Check sheet for the drawn part. Datum: minimum x, y, z corner. Units: mm. A direction names the side the tool comes from. Coordinates: 2 decimals unless noted, no trailing zeros. Write each loop counter-clockwise with the first axis right and the second up, starting at its lowest first coordinate (ties: lowest second). Pieces come first, ordered by that corner, then holes. Notation, with made-up numbers: (22.5, 63) - (66.5, 63) arc R17 ccw to (66.5, 77) - close; hole circle Ø7 at (54, 61). An arc over 180 degrees is marked (long way). Answer as CSV lines item,"result". Start each with the question number.
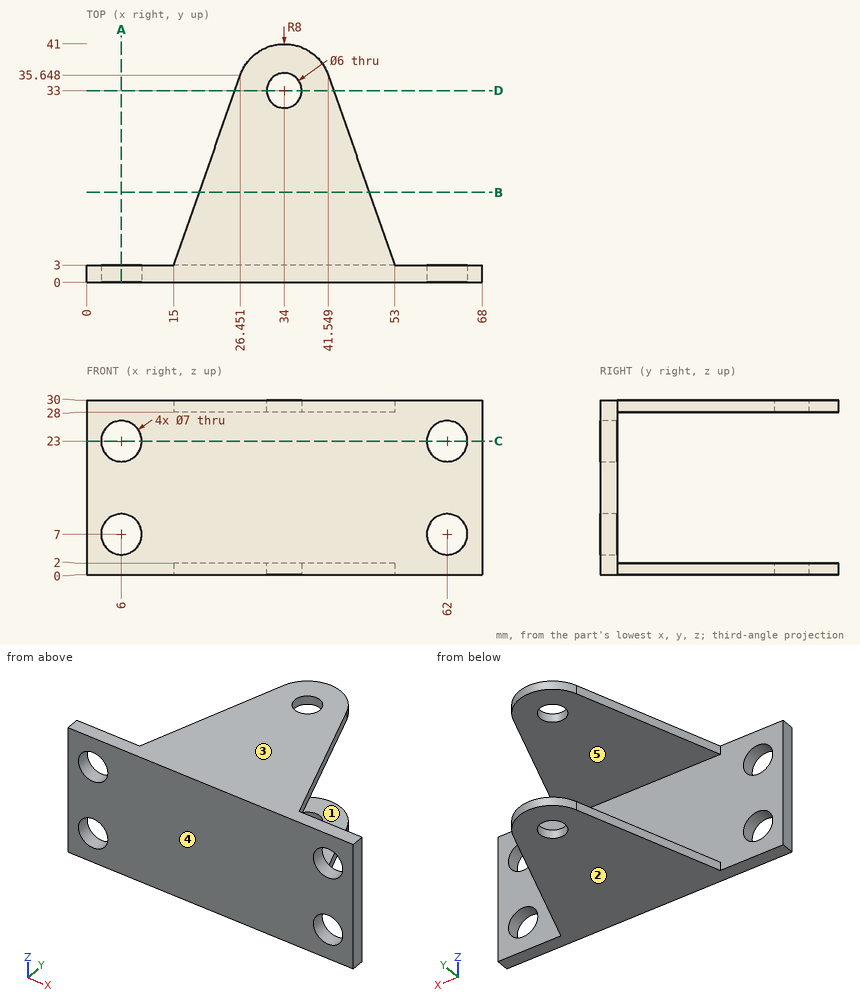
(1) Go/stop test with flat-tipped pins: P1, Ø1, axis at x = 8.5, z = 6.5, coming from the +Y side; P2, Ø8, axis at x = 62, z = 7, coming from the +Y side; P3, Ø12, axis at x = 43, z = 25.5, coming from the -Y side. Record where each tip stops, or that it passes through.
(2) Material ranges on probe 1 along X at (y, z) = (2.4, 23); probe 2 along Z at (x, y) = (30.5, 38); probe 3 along Y at (x, z) = (34, 28.4), recorded low to high. Write a range as from..to.
(3) Cross-section at D-D on y = 33. Record the boundary of the cut face in (x, z), plus the area to 3 significant figures.
(4) Cross-section at B-B on y = 15.5. Record the boundary of the cut face in (x, z).
(5) Tool access check on the marked faces 1 and 2. Record the directions out of +Z, -Z, +X, -X, +Y, -Y that give a thin tool (end or side, any length) a straight path to the whole face; none if there is none.
(6) Cross-section at C-C on z = 23. Record the boundary of the cut face in (x, y), plus the area to 3 significant figures.
(7) Cross-section at A-A on x = 6. Record the boundary of the cut face in (y, z), plus the area to 3 significant figures.
(8) Release check for a two-part mould opening along Z. For the marked faces 3, 4 and 5 record: pulls with the +Z half, pulls with the -Z half, needs draft (parallel to the pull), parting line crosses it, or undercut.
Checked values:
1,P1,"through"
1,P2,"y = 3"
1,P3,"y = 0"
2,probe 1,"0..2.5, 9.5..58.5, 65.5..68"
2,probe 2,"0..2, 28..30"
2,probe 3,"0..30, 36..41"
3,outline,"(25.52, 0) - (31, 0) - (31, 2) - (25.52, 2) - close; (25.52, 28) - (31, 28) - (31, 30) - (25.52, 30) - close; (37, 0) - (42.48, 0) - (42.48, 2) - (37, 2) - close; (37, 28) - (42.48, 28) - (42.48, 30) - (37, 30) - close"
3,area,"43.8 mm^2"
4,outline,"(19.38, 0) - (48.62, 0) - (48.62, 2) - (19.38, 2) - close; (19.38, 28) - (48.62, 28) - (48.62, 30) - (19.38, 30) - close"
5,face 1,"+X, -X, +Y"
5,face 2,"-Z, +X, -X, +Y, -Y"
6,outline,"(0, 0) - (2.5, 0) - (2.5, 3) - (0, 3) - close; (9.5, 0) - (58.5, 0) - (58.5, 3) - (9.5, 3) - close; (65.5, 0) - (68, 0) - (68, 3) - (65.5, 3) - close"
6,area,"162 mm^2"
7,outline,"(0, 0) - (3, 0) - (3, 3.5) - (0, 3.5) - close; (0, 10.5) - (3, 10.5) - (3, 19.5) - (0, 19.5) - close; (0, 26.5) - (3, 26.5) - (3, 30) - (0, 30) - close"
7,area,"48.0 mm^2"
8,face 3,"pulls with the +Z half"
8,face 4,"needs draft"
8,face 5,"undercut"
